Geometry: see drawing. Coordinates: mm, zero at the bounding-box minimum. Coordinates: 2 decimals unless noted, no trailing zeros. Write each loop counter-clockwise with the first axis right and the second up, starting at its lowest first coordinate (ties: lowest second). Pieces come first, ordered by that corner, then holes. Notation, with made-up numbers: M -2,14 L 11,14 A20 ccw 11,28 Z; hole C 86,51 d7. An arc over 180 degrees is marked long. Answer as CSV lines item,"result". Start each with the question number.
1. Line query: probe 1 along Y at (x, z) = (53.5, 15.5); probe 2 along Y at (x, z) = (113.5, 7.5) (1 decimal); probe 3 along Z at (x, y) = (31, 29.25). Output: solid intervals per line, ascending. Write a range as [from, to].
2. Contact query for flat-ended pins moving along their axis: pin 1 Ø1 at (x, y) = (91.5, 25) entering from -Z; pin 2 Ø1.9 at (x, z) = (72.5, 5) entering from +Y. Output: stop coordinate, or through.
3. Section A-A on x = 69. Return the cut outline in (y, z) (1 decimal).
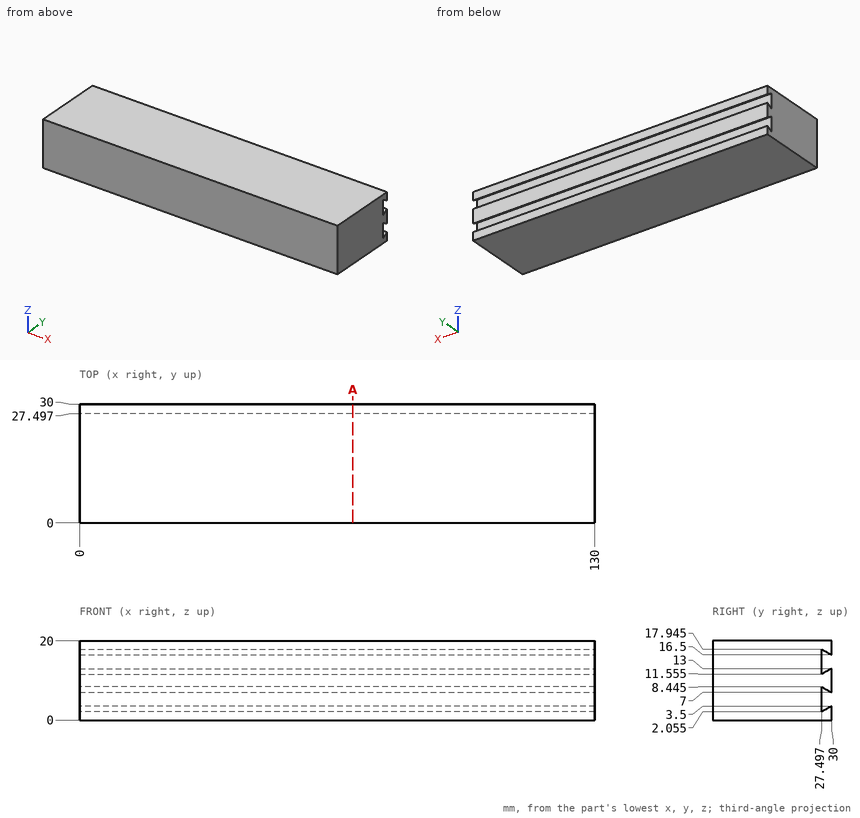
Values:
1,probe 1,"[0, 27.5]"
1,probe 2,"[0, 27.5], [29.1, 30]"
1,probe 3,"[0, 3.07], [7.43, 12.57], [16.93, 20]"
2,pin 1,"z = 0"
2,pin 2,"y = 27.5"
3,outline,"M 0,0 L 30,0 L 30,3.5 L 27.5,2.1 L 27.5,8.4 L 30,7 L 30,13 L 27.5,11.6 L 27.5,17.9 L 30,16.5 L 30,20 L 0,20 Z"
